Read the model definition and answer for the solid it produces. Units are mm, in the model's axes. A direction names the side the tool comes from. Give positions to 0.01 mm unless a question says otherwise; leave off trailing zeros. Order: outer loops, then holes, each group sorted by start corner. A loop starts at its lowest first (then second) coordinate and runs counter-clockwise, first axis right, second up.
```python
from build123d import *

# Parameters (mm, degrees)
F1_DEPTH = 63.25
F2_R     = 2
F3_DEPTH = 25


# Not quite as in the source:
# - a feature names something its author has since deleted; it is built from what else it names


with BuildPart() as f1:
    # F0 (on Top) → F1 (new body)
    with BuildSketch(Plane.XY):
        with BuildLine():
            Line((-62.75, -30.5), (-62.75, 30))
            Line((-62.75, 30), (-64.25, 30))
            Line((-64.25, 30), (-64.25, -30))
            ThreePointArc((-64.25, -30), (-62.7855339059, -33.5355339059), (-59.25, -35))
            Line((-59.25, -35), (47.75, -35))
            ThreePointArc((47.75, -35), (51.2855339059, -33.5355339059), (52.75, -30))
            Line((52.75, -30), (52.75, 30))
            ThreePointArc((52.75, 30), (51.2855339059, 33.5355339059), (47.75, 35))
            Line((47.75, 35), (-47.75, 35))
            ThreePointArc((-47.75, 35), (-51.2855339059, 33.5355339059), (-52.75, 30))
            Line((-52.75, 30), (-52.75, -1))
            Line((-52.75, -1), (-51.25, -1))
            Line((-51.25, -1), (-51.25, 30.5))
            ThreePointArc((-51.25, 30.5), (-50.3713203436, 32.6213203436), (-48.25, 33.5))
            Line((-48.25, 33.5), (48.25, 33.5))
            ThreePointArc((48.25, 33.5), (50.3713203436, 32.6213203436), (51.25, 30.5))
            Line((51.25, 30.5), (51.25, -30.5))
            ThreePointArc((51.25, -30.5), (50.3713203436, -32.6213203436), (48.25, -33.5))
            Line((48.25, -33.5), (-59.75, -33.5))
            ThreePointArc((-59.75, -33.5), (-61.8713203436, -32.6213203436), (-62.75, -30.5))
        make_face()
    extrude(amount=F1_DEPTH)

    # F2 (on face) → F3 (cut)
    with BuildSketch(Plane.XZ.offset(35)):
        with BuildLine():
            Line((21.25, 52), (-22.75, 52))
            ThreePointArc((-22.75, 52), (-24.8713203436, 51.1213203436), (-25.75, 49))
            Line((-25.75, 49), (-25.75, 17))
            ThreePointArc((-25.75, 17), (-24.8713203436, 14.8786796564), (-22.75, 14))
            Line((-22.75, 14), (21.25, 14))
            ThreePointArc((21.25, 14), (23.3713203436, 14.8786796564), (24.25, 17))
            Line((24.25, 17), (24.25, 49))
            ThreePointArc((24.25, 49), (23.3713203436, 51.1213203436), (21.25, 52))
        make_face()
        with Locations((-25.75, 58)):
            Circle(F2_R)
        with Locations((24.25, 58)):
            Circle(F2_R)
        with Locations((24.25, 8)):
            Circle(F2_R)
        with Locations((-25.75, 8)):
            Circle(F2_R)
        with BuildLine():
            ThreePointArc((-8.25, 8.5), (-7.8106601718, 7.4393398282), (-6.75, 7))
            Line((-6.75, 7), (5.25, 7))
            ThreePointArc((5.25, 7), (6.3106601718, 7.4393398282), (6.75, 8.5))
            ThreePointArc((6.75, 8.5), (6.3106601718, 9.5606601718), (5.25, 10))
            Line((5.25, 10), (-6.75, 10))
            ThreePointArc((-6.75, 10), (-7.8106601718, 9.5606601718), (-8.25, 8.5))
        make_face()
        with Locations((-19.75, 8)):
            Circle(F2_R)
        with Locations((-19.75, 58)):
            Circle(F2_R)
        with Locations((18.25, 58)):
            Circle(F2_R)
        with Locations((15.25, 8)):
            Circle(F2_R)
    extrude(amount=-F3_DEPTH, mode=Mode.SUBTRACT)


solid = f1.part
```
1) For a pull along Y with two mould halves and no side action, classify faces 4 (the face through (-50.39, 32.6, 31.18)), 5 (the face through (23.35, -34.26, 14.86)), 6 (the face through (-51.25, 33.57, 31.18)) as released by +Y, released by -Y, zero draft, split by the parting line, or undercut.
Final values:
face 4: undercut
face 5: zero draft
face 6: released by +Y
2) A tool of negligible diameter and unlimited length cuts with its end or side. For faces 1 (the face through (50.35, 32.64, 31.18)), 2 (the face through (1, 35, 31)), 3 (the face through (-26.01, -34.26, 9.983)), from which of +Z, -Z, +X, -X, +Y, -Y can it reach the whole face along a straight path? Write none if from no direction.
Final values:
face 1: +Z, -Z
face 2: +Z, -Z, +X, -X, +Y
face 3: -Y
3) The part is cut by section D-D on y = -13. Determine the outline of the cut face in (x, z), and give its area (3 significant figures).
Final values:
outline: (-64.25, 0) - (-62.75, 0) - (-62.75, 63.25) - (-64.25, 63.25) - close; (51.25, 0) - (52.75, 0) - (52.75, 63.25) - (51.25, 63.25) - close
area: 190 mm2
4) The part is cut by section A-A on x = 35. Determine the outline of the cut face in (y, z).
Final values:
outline: (-35, 0) - (-33.5, 0) - (-33.5, 63.25) - (-35, 63.25) - close; (33.5, 0) - (35, 0) - (35, 63.25) - (33.5, 63.25) - close
5) Consider L1, parallel to Z at x = 15.25, y = -34.1; L2, parallel to X at y = 14.5, z = 43; L3, parallel to Z at x = -19.75, y = -34.6. Determine where each line is inside the solid, lowest interval first.
Final values:
L1: z = 0 to 6, 10 to 14, 52 to 63.25
L2: x = -64.25 to -62.75, -52.75 to -51.25, 51.25 to 52.75
L3: z = 0 to 6, 10 to 14, 52 to 56, 60 to 63.25
6) Given pin 1 (3.5 mm diameter, centred on x = -25.75, z = 8, fed in from -Y); pin 2 (1.2 mm diameter, centred on y = -34, z = 32, fed in from +X); pin 3 (1.5 mm diameter, centred on x = -50.5, z = 35, fed in from +Y); pin 4 (12 mm diameter, centred on x = -20.5, y = -27, fed in from +Z), each flat-ended and moving along its own axis, determine where each tip first touches the part or whether it passes through.
Final values:
pin 1: stops at y = 33.5
pin 2: stops at x = 51.42
pin 3: stops at y = 34.58
pin 4: passes through
7) The part is cut by section C-C on x = -11. Determine the outline of the cut face in (y, z).
Final values:
outline: (-35, 0) - (-33.5, 0) - (-33.5, 14) - (-35, 14) - close; (-35, 52) - (-33.5, 52) - (-33.5, 63.25) - (-35, 63.25) - close; (33.5, 0) - (35, 0) - (35, 63.25) - (33.5, 63.25) - close
8) The part is cut by section B-B on z = 24. Determine the outline of the cut face in (x, y).
Final values:
outline: (-64.25, -30) arc R5 ccw to (-59.25, -35) - (-25.75, -35) - (-25.75, -33.5) - (-59.75, -33.5) arc R3 cw to (-62.75, -30.5) - (-62.75, 30) - (-64.25, 30) - close; (-52.75, -1) - (-51.25, -1) - (-51.25, 30.5) arc R3 cw to (-48.25, 33.5) - (48.25, 33.5) arc R3 cw to (51.25, 30.5) - (51.25, -30.5) arc R3 cw to (48.25, -33.5) - (24.25, -33.5) - (24.25, -35) - (47.75, -35) arc R5 ccw to (52.75, -30) - (52.75, 30) arc R5 ccw to (47.75, 35) - (-47.75, 35) arc R5 ccw to (-52.75, 30) - close
